Could you check a few things on this model? Use its own coordinates, in mm. A direction names the side the tool comes from. Coordinates: 2 decimals unless noted, no trailing zeros. Order: outer loops, then holes, each group sorted by start corner. A loop starts at its lowest first (then second) coordinate and runs counter-clockwise, first axis right, second up. Notation, with made-up numbers: (87, 13) -> (115, 13) arc R28 cw to (115, 51) -> close; hole circle Ø5 at (-12, 71.25). An arc over 180 degrees is marked (long way). Put each result on its own line as item: value. Start each with the question number.
Q1. For faces 5 (the face through (10, 0, -227)), 6 (the face through (-187, -29, -111)), 7 (the face through (1.08, -4.88, -227.46)), 8 (the face through (-190, -31, -111)), 9 (the face through (-177, 0, -215)), which set-ups out of +Z, -Z, +X, -X, +Y, -Y let a thin tool reach every point of the face, with its end or its side?
Q2. If we section it at B-B (y = -23): Please give me the cut outline in (x, z), and give its area (3 significant figures).
Q3. Please list where these lines run through material, in increasing order: line 1 along Z through (x, y) = (-99, 7.5); line 2 along X through (y, z) = (-19, -50.5); line 3 along Y through (x, z) = (7, 1.4).
Q4. If we section it at A-A (x = -113): Please give me the cut outline in (y, z).
Q5. If we section it at C-C (z = -26): Please give me the cut outline in (x, y), and give its area (3 significant figures).
Q6. Will these pins go through, and if not, where does the flat tip stop? pin 1 (12 mm diameter, centred on x = -167, y = -20.5, fed in from +Z); pin 2 (2.5 mm diameter, centred on x = 0, y = 7, fed in from +Z); pin 3 (24 mm diameter, centred on y = -26.5, z = -147.5, fed in from +X); pin 4 (1.5 mm diameter, centred on x = -188, y = -32, fed in from +Z).
Q7. We'd pull the mould along Z, two halves only. Please class faces 1 (the face through (10, 0, 2)), 2 (the face through (-91, 0, 5)), 3 (the face through (-89, 0, -230)), 4 (the face through (-177, 0, -10)): +Z half, -Z half, draft (parallel to the pull), parting line (faces both ways), or undercut.
from build123d import *

# Parameters (mm, degrees)
SKETCH_1_R      = 1.5
EXTRUDE_1_DEPTH = 5
EXTRUDE_2_DEPTH = 225
RIB_1_REACH     = 307.164
SKETCH_3_WALL_W = 640.612052034
SKETCH_3_WALL_H = 20
SKETCH_4_R      = 5
EXTRUDE_3_DEPTH = 5


with BuildPart() as part:
    # 草图1 → 凸台-拉伸1 (new body)
    with BuildSketch(Plane.XY):
        with BuildLine():
            Line((0, 10), (-190, 10))
            Line((-190, 10), (-190, -10))
            Line((-190, -10), (0, -10))
            ThreePointArc((0, -10), (10, 0), (0, 10))
        make_face()
        with Locations((7, 0)):
            Circle(SKETCH_1_R, mode=Mode.SUBTRACT)
        with Locations((0, -7)):
            Circle(SKETCH_1_R, mode=Mode.SUBTRACT)
        with Locations((-7, 0)):
            Circle(SKETCH_1_R, mode=Mode.SUBTRACT)
        with Locations((0, 7)):
            Circle(SKETCH_1_R, mode=Mode.SUBTRACT)
    extrude(amount=EXTRUDE_1_DEPTH)

    # 草图2 → 凸台-拉伸2 (add)
    with BuildSketch(Plane(origin=(0, 0, 0), x_dir=(-1, 0, 0), z_dir=(0, 0, -1))):
        Polygon((190, 10), (190, -10), (190, -70), (187, -70), (187, -10), (187, 10), align=None)
    extrude(amount=EXTRUDE_2_DEPTH)

    # 草图3 wall → 筋1 (add, up to next)
    with BuildSketch(Plane(origin=(-177, 10, -10), x_dir=(0.707106781187, 0, 0.707106781187), z_dir=(0.707106781187, 0, -0.707106781187)), mode=Mode.PRIVATE) as rib_1_sk1:
        with Locations((0, 10)):
            Rectangle(SKETCH_3_WALL_W, SKETCH_3_WALL_H)
    rib_1_tool1 = extrude(rib_1_sk1.sketch, amount=-RIB_1_REACH, mode=Mode.PRIVATE) - part.part
    rib_1 = rib_1_tool1.solids().sort_by_distance((-177, 10, -10))[0]
    add(rib_1)

    # 草图4 → 凸台-拉伸3 (add)
    with BuildSketch(Plane(origin=(0, 0, -225), x_dir=(-1, 0, 0), z_dir=(0, 0, -1))):
        with BuildLine():
            Line((190, -10), (190, 10))
            Line((190, 10), (0, 10))
            ThreePointArc((0, 10), (-10, 0), (0, -10))
            Line((0, -10), (190, -10))
        make_face()
        Circle(SKETCH_4_R, mode=Mode.SUBTRACT)
    extrude(amount=EXTRUDE_3_DEPTH)

    # 镜向1: 筋1 across plane
    add(rib_1.mirror(Plane.XY.offset(-112.5)))


solid = part.part
The answers:
1. face 5: +Z, -Z, +X
1. face 6: +X, -Y
1. face 7: -Z
1. face 8: +Z, -Z, -X, +Y, -Y
1. face 9: +X, +Y, -Y
2. outline: (-190, -225) -> (-187, -225) -> (-187, 0) -> (-190, 0) -> close
2. area: 675 mm^2
3. line 1: -230 to -225, 0 to 5
3. line 2: -190 to -187
3. line 3: -7.14 to -1.5, 1.5 to 7.14
4. outline: (-10, -230) -> (10, -230) -> (10, -225) -> (-10, -225) -> close; (-10, 0) -> (10, 0) -> (10, 5) -> (-10, 5) -> close
5. outline: (-190, -70) -> (-187, -70) -> (-187, 10) -> (-190, 10) -> close
5. area: 240 mm^2
6. pin 1: through
6. pin 2: z = -225
6. pin 3: x = -187
6. pin 4: z = 0
7. face 1: draft
7. face 2: +Z half
7. face 3: -Z half
7. face 4: undercut
